```python
from build123d import *

# Parameters (mm, degrees)
F1_DEPTH = 60.198
F2_DEPTH = 60.198
F0_W     = 10.922
F0_H     = 33.528
F3_DEPTH = 50.8
F4_DEPTH = 10.922
F5_R     = 7.874
F6_DEPTH = 10.923
F7_DEPTH = 25.4
F9_DEPTH = 25.4


with BuildPart() as f1:
    # F0 (on Top) → F1 (new body)
    with BuildSketch(Plane.XY):
        Polygon((-70.913484, -4.775751), (-81.835484, -4.775751), (-81.835484, -15.697751), (-70.913484, -15.697751), (-50.085484, -15.697751), (-50.085484, -4.775751), align=None)
    extrude(amount=F1_DEPTH)

    # F0 (on Top) → F2 (join)
    with BuildSketch(Plane.XY):
        Polygon((32.464516, -4.775751), (-50.085484, -4.775751), (-50.085484, -15.697751), (-7.413484, -15.697751), (32.464516, -15.697751), align=None)
    extrude(amount=F2_DEPTH)

    # F0 (on Top) → F3 (join)
    with BuildSketch(Plane.XY):
        with Locations((-76.374484, -32.461751)):
            Rectangle(F0_W, F0_H)
    extrude(amount=F3_DEPTH)

    # F0 (on Top) → F4 (join)
    with BuildSketch(Plane.XY):
        Polygon((-50.085484, -15.697751), (-70.913484, -15.697751), (-70.913484, -49.225751), (-7.413484, -15.697751), align=None)
    extrude(amount=F4_DEPTH)

    # F5 (on face) → F6 (cut, through all)
    with BuildSketch(Plane.XZ.offset(15.697751)):
        with Locations((13.414516, 19.05)):
            Circle(F5_R)
    extrude(amount=-F6_DEPTH, mode=Mode.SUBTRACT)

    # F5 (on face) → F7 (cut)
    with BuildSketch(Plane.XZ.offset(15.697751)):
        Polygon((32.464516, 60.198), (-50.085484, 60.198), (32.464516, 40.890517), align=None)
    extrude(amount=-F7_DEPTH, mode=Mode.SUBTRACT)

    # F8 (on face) → F9 (cut)
    with BuildSketch(Plane(origin=(-81.835484, 0, 0), x_dir=(0, -1, 0), z_dir=(-1, 0, 0))):
        Polygon((49.225751, 50.8), (32.461751, 50.8), (49.225751, 22.098), align=None)
    extrude(amount=-F9_DEPTH, mode=Mode.SUBTRACT)


solid = f1.part
```
Input: part model. Units: mm. Frame: model coordinates. A direction names the side the tool comes from. Give positions to 0.01 mm unless a question says otherwise; leave off trailing zeros. Order: outer loops, then holes, each group sorted by start corner. A loop starts at its lowest first (then second) coordinate and runs counter-clockwise, first axis right, second up. Notation, with made-up numbers: (76, 73.25) - (119, 73.25) arc R17 cw to (119, 102.25) - close; hole circle Ø11 at (-29, 30.25). An arc over 180 degrees is marked (long way). One line per item, written item: value.
1. Reachability of faces 1 (the face through (-81.835, -22, 23)), 2 (the face through (-70.913, -29, 31)), 3 (the face through (-76, -24, 50.8)) from +Z, -Z, +X, -X, +Y, -Y: full face, straight path, thin tool, end or side. Return the list, or none.
Determined:
face 1: +Z, -Z, -X, +Y, -Y
face 2: +Z, +X, -Y
face 3: +Z, +X, -X, -Y
2. Cut plane A-A, the plane z = 19.05. Output: boundary loops of the cut face in (x, y), and give its area (3 significant figures).
Determined:
outline: (-81.84, -49.23) - (-70.91, -49.23) - (-70.91, -15.7) - (5.54, -15.7) - (5.54, -4.78) - (-81.84, -4.78) - close; (21.29, -15.7) - (32.46, -15.7) - (32.46, -4.78) - (21.29, -4.78) - close
area: 1,440 mm2
3. Draft query along Z for faces 4 (the face through (32.465, -10, 20)), 5 (the face through (11.708, -10.313, 11.363)), 6 (the face through (-66, -10, 60.198)). Return one class per face: released by +Z, released by -Z, zero draft, split by the parting line, or undercut.
Determined:
face 4: zero draft
face 5: undercut
face 6: released by +Z
4. Cut plane B-B, the plane y = -19.5. Output: boundary loops of the cut face in (x, z), and give its area (3 significant figures).
Determined:
outline: (-81.84, 0) - (-14.61, 0) - (-14.61, 10.92) - (-70.91, 10.92) - (-70.91, 50.8) - (-81.84, 50.8) - close
area: 1,170 mm2
5. Cut plane C-C, the plane x = -57. Output: boundary loops of the cut face in (y, z).
Determined:
outline: (-41.88, 0) - (-4.78, 0) - (-4.78, 60.2) - (-15.7, 60.2) - (-15.7, 10.92) - (-41.88, 10.92) - close
6. Line query: probe 1 along X at (y, z) = (-10, 19); probe 2 along Z at (x, y) = (-58, -24); probe 3 along Y at (x, z) = (-28.5, 43.5). Output: solid intervals per line, ascending.
Determined:
probe 1: -81.84 to 5.54, 21.29 to 32.46
probe 2: 0 to 10.92
probe 3: -15.7 to -4.78
7. Pin query (flat end, axial travel): pin 1 Ø6 at (y, z) = (-39.5, 41) entering from +X; pin 2 Ø3.5 at (x, y) = (-77, -24) entering from +Z; pin 3 Ø14 at (x, z) = (13.41, 19.05) entering from +Y; pin 4 Ø4 at (x, y) = (-55.5, -30.5) entering from +Z. Return the tip coordinate at first contact, or that it passes through.
Determined:
pin 1: x = -70.91
pin 2: z = 50.8
pin 3: through
pin 4: z = 10.92
8. Cut plane D-D, the plane x = 3.5. Output: boundary loops of the cut face in (y, z).
Determined:
outline: (-15.7, 0) - (-4.78, 0) - (-4.78, 47.66) - (-15.7, 47.66) - close
